The listing builds one solid part. Answer for the finished solid, in the listing's coordinates (mm). A direction names the side the tool comes from. Coordinates: 2 decimals unless noted, no trailing zeros. Order: outer loops, then holes, each group sorted by start corner. A loop starts at its lowest first (then second) coordinate and runs counter-clockwise, first axis right, second up.
from build123d import *

# Parameters (mm, degrees)
ESQUISSE1_W             = 12
ESQUISSE1_H             = 10.5
BOSS_EXTRU_1_DEPTH      = 16.2
ENL_V_MAT_EXTRU_1_DEPTH = 14
ESQUISSE3_W             = 5
ESQUISSE3_H             = 2.5
BOSS_EXTRU_2_DEPTH      = 16


with BuildPart() as part:
    # Esquisse1 → Boss.-Extru.1 (new body)
    with BuildSketch(Plane.XY):
        Rectangle(ESQUISSE1_W, ESQUISSE1_H)
    extrude(amount=-BOSS_EXTRU_1_DEPTH)

    # Esquisse2 → Enlèv. mat.-Extru.1 (cut)
    with BuildSketch(Plane.XY):
        Polygon((-5, 1), (-2.5, 4), (2.5, 4), (5, 1), (5, -4), (-5, -4), align=None)
    extrude(amount=-ENL_V_MAT_EXTRU_1_DEPTH, mode=Mode.SUBTRACT)

    # Esquisse3 → Boss.-Extru.2 (add)
    with BuildSketch(Plane(origin=(0, 0, -16.2), x_dir=(-1, 0, 0), z_dir=(0, 0, -1))):
        Rectangle(ESQUISSE3_W, ESQUISSE3_H)
    extrude(amount=-BOSS_EXTRU_2_DEPTH)


solid = part.part
1) Section B-B (x = -3.5) is taken. Give the vertices of the cut face in (y, z), then the cut area to 3 significant figures.
2) Section A-A (z = -11.5) is taken. Give the vertices of the cut face in (x, y).
3) Section C-C (y = -2) is taken. Give the vertices of the cut face in (x, z).
4) Section D-D (x = 1.25) is taken. Give the vertices of the cut face in (y, z), then the cut area to 3 significant figures.
5) Determine the mould class of faces 3 (the face through (3.732, 2.521, -6.902)), 4 (the face through (6, 0, -8)), 5 (the face through (-6, 0, -8)), 6 (the face through (0, 0, -16.2)) for opening direction X: released by +X, released by -X, zero draft, split by the parting line, or undercut.
6) A tool of negligible diameter and unlimited length cuts with its end or side. For faces 1 (the face through (5, -1, -7)), 2 (the face through (0, 5.25, -8)), from which of +Z, -Z, +X, -X, +Y, -Y can it reach the whole face along a straight path? Write none if from no direction.
7) Consider L1, parallel to Y at x = -1.75, z = -7.5; L2, parallel to X at y = 0, z = -2.5; L3, parallel to X at y = -1.75, z = -5.75. Determine where each line is inside the solid, lowest interval first.
8) This flat-tipped pin is pushed along its axis until it touches: P1, Ø0.8, axis at x = -0.5, y = 0, coming from the +Z side. Where does it stop, or does it pass through?
Filled sheet:
1. outline: (-5.25, -16.2) - (5.25, -16.2) - (5.25, 0) - (2.8, 0) - (2.8, -14) - (-4, -14) - (-4, 0) - (-5.25, 0) - close
1. area: 74.9 mm2
2. outline: (-6, -5.25) - (6, -5.25) - (6, 5.25) - (-6, 5.25) - close; (-2.5, -1.25) - (2.5, -1.25) - (2.5, 1.25) - (-2.5, 1.25) - close; hole (-5, -4) - (5, -4) - (5, 1) - (2.5, 4) - (-2.5, 4) - (-5, 1) - close
3. outline: (-6, -16.2) - (6, -16.2) - (6, 0) - (5, 0) - (5, -14) - (-5, -14) - (-5, 0) - (-6, 0) - close
4. outline: (-5.25, -16.2) - (5.25, -16.2) - (5.25, 0) - (4, 0) - (4, -14) - (1.25, -14) - (1.25, -0.2) - (-1.25, -0.2) - (-1.25, -14) - (-4, -14) - (-4, 0) - (-5.25, 0) - close
4. area: 92.6 mm2
5. face 3: undercut
5. face 4: released by +X
5. face 5: released by -X
5. face 6: zero draft
6. face 1: +Z
6. face 2: +Z, -Z, +X, -X, +Y
7. L1: y = -5.25 to -4, -1.25 to 1.25, 4 to 5.25
7. L2: x = -6 to -5, -2.5 to 2.5, 5 to 6
7. L3: x = -6 to -5, 5 to 6
8. P1: stops at z = -0.2
